Build history of the part. All positions in model axes, mm. A direction names the side the tool comes from. Give positions to 0.01 mm unless a question says otherwise; leave off trailing zeros. Order: outer loops, then holes, each group sorted by start corner. A loop starts at its lowest first (then second) coordinate and runs counter-clockwise, first axis right, second up. Notation, with made-up numbers: (13, 46) - (32, 46) arc R24 cw to (32, 72) - close; hole circle Ø10 at (-10, 81.25). An arc over 180 degrees is marked (long way). Answer in a Markdown table with one row per item.
```python
from build123d import *

# Parameters (mm, degrees)
SKETCH1_R           = 4.7625
BOSS_EXTRUDE1_DEPTH = 31.75
SKETCH2_R           = 2.4892
CUT_EXTRUDE1_DEPTH  = 25.4
SKETCH3_W           = 64.987057328
SKETCH3_H           = 9.244924149
SKETCH3_W_2         = 60.957372158
SKETCH3_H_2         = 11.477125068
CUT_EXTRUDE2_DEPTH  = 32.7500001
FILLET1_R           = 2.54
FILLET2_R           = 12.7


with BuildPart() as part:
    # Sketch1 → Boss-Extrude1 (new body)
    with BuildSketch(Plane.XY):
        with BuildLine():
            Line((-12.474995441, -32.621007246), (-17.01135742, -44.483191699))
            ThreePointArc((-17.01135742, -44.483191699), (4.857819156, -83.447185108), (-29.486352861, -112.029198945))
            Line((-29.486352861, -112.029198945), (-29.486352861, -117.566398945))
            Line((-29.486352861, -117.566398945), (17.033444212, -117.566398945))
            Line((17.033444212, -117.566398945), (71.902434201, -53.852584939))
            ThreePointArc((71.902434201, -53.852584939), (74.265423414, -49.285430405), (74.319342365, -44.143474424))
            Line((74.319342365, -44.143474424), (55.334619846, 39.5732))
            Line((55.334619846, 39.5732), (0, 39.5732))
            Line((0, 39.5732), (0, 34.925))
            ThreePointArc((0, 34.925), (34.344172017, -6.342986163), (-12.474995441, -32.621007246))
        make_face()
        with Locations((18.773647139, -98.516398945)):
            Circle(SKETCH1_R, mode=Mode.SUBTRACT)
        with BuildLine():
            ThreePointArc((4.805346172, -54.132368316), (4.611000081, -47.373075962), (10.619637037, -44.271127306))
            Line((10.619637037, -44.271127306), (48.106372009, -47.462477992))
            ThreePointArc((48.106372009, -47.462477992), (51.235190632, -48.60574982), (53.354739272, -51.17559223))
            ThreePointArc((53.354739272, -51.17559223), (54.288815903, -52.843916254), (55.495053497, -54.327423945))
            ThreePointArc((55.495053497, -54.327423945), (57.278420501, -58.558773894), (55.742748768, -62.886178727))
            Line((55.742748768, -62.886178727), (33.730414898, -88.446877882))
            ThreePointArc((33.730414898, -88.446877882), (29.678710415, -90.607528488), (25.229617999, -89.471616111))
            ThreePointArc((25.229617999, -89.471616111), (21.919602705, -87.858508918), (18.264177504, -87.415583797))
            ThreePointArc((18.264177504, -87.415583797), (13.399411545, -85.477293546), (11.645131351, -80.543185934))
            ThreePointArc((11.645131351, -80.543185934), (10.470460882, -66.756317013), (4.805346172, -54.132368316))
        make_face(mode=Mode.SUBTRACT)
        with Locations((63.482010487, -46.601094008)):
            Circle(SKETCH1_R, mode=Mode.SUBTRACT)
        with BuildLine():
            Line((49.704289076, -41.541119878), (33.019297292, -40.120679821))
            ThreePointArc((33.019297292, -40.120679821), (27.589635384, -35.961933342), (29.083549865, -29.28775772))
            ThreePointArc((29.083549865, -29.28775772), (38.598079931, -14.622374999), (41.18881011, 2.665998258))
            ThreePointArc((41.18881011, 2.665998258), (42.985049027, 7.515335292), (47.792622808, 9.420532987))
            ThreePointArc((47.792622808, 9.420532987), (48.759316239, 9.421923517), (49.722231073, 9.507323433))
            ThreePointArc((49.722231073, 9.507323433), (54.184633542, 8.424879689), (56.750552758, 4.616890871))
            Line((56.750552758, 4.616890871), (64.280599338, -28.588253807))
            ThreePointArc((64.280599338, -28.588253807), (63.608310734, -33.130582317), (60.049355437, -36.032057365))
            ThreePointArc((60.049355437, -36.032057365), (57.324876061, -37.350291237), (55.057143591, -39.354765694))
            ThreePointArc((55.057143591, -39.354765694), (52.644006558, -41.092556671), (49.704289076, -41.541119878))
        make_face(mode=Mode.SUBTRACT)
        with Locations((48.26, 20.5232)):
            Circle(SKETCH1_R, mode=Mode.SUBTRACT)
    extrude(amount=BOSS_EXTRUDE1_DEPTH)

    # Sketch2 → Cut-Extrude1 (cut)
    with BuildSketch(Plane(origin=(0, 0, 0), x_dir=(0, 0, 1), z_dir=(-0.934030272, 0.357193857, 0))):
        with Locations((7.9375, -41.275)):
            Circle(SKETCH2_R)
        with Locations((23.8125, -41.275)):
            Circle(SKETCH2_R)
    extrude(amount=-CUT_EXTRUDE1_DEPTH, mode=Mode.SUBTRACT)

    # Sketch3 → Cut-Extrude2 (cut, through all)
    with BuildSketch(Plane.XY.offset(31.75)):
        Polygon((-17.01135742, -44.483191699), (-12.474995441, -32.621007246), (-5.676500584, -32.621007246), (-11.862088463, -48.795771234), align=None)
        with Locations((32.493528664, 39.547462075)):
            Rectangle(SKETCH3_W, SKETCH3_H)
        with Locations((0.992333218, -117.767761479)):
            Rectangle(SKETCH3_W_2, SKETCH3_H_2)
    extrude(amount=-CUT_EXTRUDE2_DEPTH, mode=Mode.SUBTRACT)

    # Fillet1
    fillet1_edges = [part.edges().sort_by_distance(p)[0] for p in [
        (-29.486352861, -112.029198945, 15.875),
        (0, 34.925, 15.875),
    ]]
    fillet(fillet1_edges, radius=FILLET1_R)

    # Fillet2
    fillet2_edges = [part.edges().sort_by_distance(p)[0] for p in [
        (56.388708387, 34.925, 15.875),
        (21.801963819, -112.029198945, 15.875),
    ]]
    fillet(fillet2_edges, radius=FILLET2_R)


solid = part.part
```
1. Drop flat-ended pins along their axis: P1, Ø11, axis at x = 18.77, y = -98.52, coming from the -Z side; P2, Ø4, axis at y = -80.5, z = 22, coming from the -X side; P3, Ø3, axis at y = -26.5, z = 22.5, coming from the +X side; P4, Ø4, axis at y = -64, z = 17.5, coming from the -X side. Give the stop position or say it passes through.
Check result:
| item | result |
|---|---|
| P1 | stops at z = 0 |
| P2 | stops at x = 5.02 |
| P3 | stops at x = 70.66 |
| P4 | stops at x = 2 |
2. Probe line 1 (Y direction, x = 28, z = 28) (3 decimals); line 2 (Y direction, x = 46.5, z = 14); line 3 (Y direction, x = 27, z = 12) (3 decimals). List the from-to ranges inside material, lowest first.
Check result:
| item | result |
|---|---|
| line 1 | y = -104.832 to -90.586, -45.751 to -36.865, -30.722 to -20.875, 20.875 to 34.925 |
| line 2 | y = -83.35 to -73.62, -47.33 to -41.27, 9.34 to 16.1, 24.95 to 34.92 |
| line 3 | y = -105.993 to -90.356, -45.666 to -22.153, 22.153 to 34.925 |
3. Cut at A-A on x = 66. Write the cut outline in (y, z).
Check result:
| item | result |
|---|---|
| outline | (-60.71, 0) - (-50.64, 0) - (-50.64, 31.75) - (-60.71, 31.75) - close; (-42.56, 0) - (-7.46, 0) - (-7.46, 31.75) - (-42.56, 31.75) - close |
4. Cut at C-C on x = -1. Count the separate pieces of the cut face and the enclosed holes in it, and give its area (3 significant figures).
Check result:
| item | result |
|---|---|
| separate pieces | 2 |
| enclosed holes | 2 |
| area | 1,120 mm² |
5. Which spindle directions (+Z, -Z, +X, -X, +Y, -Y) get a long thin tool onto all of the face, cutting with end or side? Do faces 5 (the face through (5.44, -76.97, 15.65)), 6 (the face through (21.969, -87.873, 15.653)). Say none if no direction does.
Check result:
| item | result |
|---|---|
| face 5 | +Z, -Z, -X |
| face 6 | +Z, -Z |
6. Two-plate mould, pull along Y, no slides. Class faces 1 (the face through (-13.089, -110.195, 16.097)), 2 (the face through (34, -44, 0)), 3 (the face through (29.101, -45.844, 15.653)), 4 (the face through (54.08, 32.22, 16.1)): +Y half, -Y half, draft (parallel to the pull), parting line (faces both ways), or undercut.
Check result:
| item | result |
|---|---|
| face 1 | parting line |
| face 2 | draft |
| face 3 | undercut |
| face 4 | +Y half |
7. Cut at B-B on y = -95.5. Write the cut outline in (x, z).
Check result:
| item | result |
|---|---|
| outline | (0.2, 0) - (15.09, 0) - (15.09, 31.75) - (0.2, 31.75) - close; (22.46, 0) - (36.04, 0) - (36.04, 31.75) - (22.46, 31.75) - close |
